Could you check a few things on this model? Use its own coordinates, in mm. Face numbers are marked on the shaded views. A direction names the side the tool comes from. Give positions to 0.01 mm unless a question says otherwise; leave off trailing zeros. Write each loop counter-clockwise with the first axis right and the second up, starting at its lowest first coordinate (ties: lowest second). Pieces come first, ordered by that corner, then holes. Notation, with made-up numbers: M 36,22.5 L 84,22.5 A14 ccw 84,48.5 Z; hole C 60,69 d9. An arc over 180 degrees is marked long. Use one line per item in the form item = value.
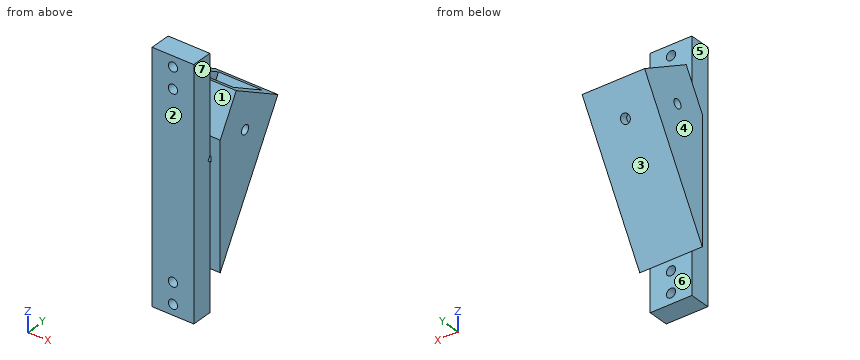
Autodesk Inventor part; units mm, degrees
ref_plane "YZ Plane" through (0, 0, 0) normal (1, 0, 0) x (0, 1, 0)
ref_plane "XZ Plane" through (0, 0, 0) normal (0, 1, 0) x (-1, 0, 0)
ref_plane "XY Plane" through (0, 0, 0) normal (0, 0, 1) x (1, 0, 0)
sketch "Sketch1" plane through (0, 0, 0) normal (1, 0, 0) x (0, 1, 0)
  line L0 (0, 0) -> (12.7, 21.997)
  line L1 (0, 0) -> (0, 47.397)
  line L2 (0, 0) -> (0, -101.6)
  line L3 (12.7, 21.997) -> (45.6956, 2.947)
  line L4 (45.6956, 2.947) -> (0, -76.2)
  line L5 (12.7, 21.997) -> (0, 21.997) construction
  line L6 (0, 47.397) -> (-12.7, 47.397)
  line L7 (-12.7, 47.397) -> (-12.7, -76.2)
  line L8 (0, -101.6) -> (-12.7, -101.6)
  line L9 (-12.7, -101.6) -> (-12.7, -76.2)
  dimension "d0" = 38.1
  dimension "d1" = 25.4
  dimension "d6" = 30
  dimension "d7" = 25.4
  dimension "d21" = 25.4
  dimension "d22" = 12.7
extrude "Extrusion2" add sketch "Sketch1" along normal mid plane 38.1 contours L0 L3 L4 L2
extrude "Extrusion3" add sketch "Sketch1" along normal mid plane 25.4
sketch "Sketch2" plane through (-19.05, 12.7, 21.997) normal (0, 0.5, 0.8660254) x (1, 0, 0)
  line L0 (32.385, 5.715) -> (32.385, 32.385)
  line L1 (32.385, 32.385) -> (5.715, 32.385)
  line L2 (5.715, 32.385) -> (5.715, 5.715)
  line L3 (5.715, 5.715) -> (32.385, 5.715)
  line L4 (32.385, 5.715) -> (5.715, 32.385) construction
  line L5 (32.385, 32.385) -> (5.715, 5.715) construction
  line L6 (0, 0) -> (0, 38.1)
  line L7 (38.1, 38.1) -> (38.1, 0)
  line L8 (0, 38.1) -> (38.1, 38.1)
  point P0 (19.05, 0)
  point P1 (19.05, 19.05)
  dimension "d16" = 26.67
  dimension "d17" = 19.05
  dimension "d18" = 19.05
extrude "Extrusion4" cut sketch "Sketch2" against normal blind 38.1
sketch "Sketch3" plane through (-12.7, 0, 47.397) normal (0, 1, 0) x (1, 0, 0)
  point P0 (12.7, 47.397)
sketch "Sketch4" plane through (-12.7, 0, 47.397) normal (0, 1, 0) x (1, 0, 0)
  line L0 (25.4, 0) -> (0, 0)
  line L1 (-6.35, 25.4) -> (31.75, 25.4)
  line L2 (0, 123.597) -> (25.4, 123.597)
  line L3 (25.4, 148.997) -> (0, 148.997)
  point P0 (12.7, 47.397)
  point P1 (12.7, 6.35)
  point P2 (12.7, 19.05)
  point P3 (12.7, 129.947)
  point P4 (12.7, 142.647)
  dimension "d23" = 6.35
  dimension "d24" = 6.35
  dimension "d25" = 6.35
  dimension "d26" = 6.35
hole "Hole1" at (0, 0, 41.047) at (0, 0, 28.347) at (0, 0, -82.55) at (0, 0, -95.25) direction (0, -1, 0) diameter 5.6134 end through all
sketch "Sketch5" plane through (19.05, 0, 0) normal (1, 0, 0) x (0, 0, -1)
  line L0 (-21.997, 12.7) -> (-2.947, 45.6956) construction
  line L1 (-12.472, 29.1978) -> (38.1, 0) construction
  line L2 (0, 0) -> (76.2, 0) construction
  line L3 (-21.997, 12.7) -> (0, 0) construction
  point P0 (4.0257, 19.6728)
  dimension "d34" = 19.05
sketch "Sketch6" plane through (-19.05, 45.6956, 2.947) normal (0, 0.8660254, -0.5) x (1, 0, 0)
  line L0 (0, 0) -> (38.1, 0)
  point P0 (19.05, 25.4)
  point P1 (19.05, 19.05)
  dimension "d35" = 19.05
hole "Hole2" at (0, 36.1706, -13.5507) direction (0, -0.8660254, 0.5) diameter 5.6134 depth 5.715
hole "Hole3" at (19.05, 19.6728, -4.0257) direction (-1, 0, 0) diameter 5.6134 end through all
properties part number "30degreeAttachement" material "PBT Plastic"
1) I want a section at C-C, the plane x = 0. Count the separate pieces of the cut face and the enclosed holes in it, plus the area to 3 significant figures.
Checked values:
separate_pieces = 6
enclosed_holes = 0
area = 2,780 mm2
2) I want a section at A-A, the plane z = -95.25. Please give me the cut outline in (x, y), plus the area to 3 significant figures.
Checked values:
outline = M -12.7,-12.7 L -2.81,-12.7 L -2.81,0 L -12.7,0 Z; M 2.81,-12.7 L 12.7,-12.7 L 12.7,0 L 2.81,0 Z
area = 251 mm2
3) For the marked faces 5, 6 and 7, which set-ups out of +Z, -Z, +X, -X, +Y, -Y let a thin tool reach every point of the face, with its end or its side?
Checked values:
face_5 = +Z, -Z, -X, -Y
face_6 = -Z, +X, -X, +Y
face_7 = +Z, -Z, +X, -Y
4) For pin 1 Ø5 at (x, z) = (-16, -26.5) entering from -Y; pin 2 Ø3 at (x, z) = (-13, -86) entering from +Y; pin 3 Ø2 at (x, y) = (-10, 6.5) entering from -Z; pin 4 Ø5 at (x, z) = (0, 41.047) entering from -Y, each with a flat end and sliding along its axis, tell me the tip position at first contact or that it passes through.
Checked values:
pin_1 = 0
pin_2 = 0
pin_3 = -66.67
pin_4 = through
5) If I drill on L1, parallel to Z at x = 0, y = -5.5; L2, parallel to X at y = 12.5, z = 6 (3 decimals); L3, parallel to Y at x = -12, z = 26, over which ranges is the centre line in solid material (lowest first)?
Checked values:
L1 = -101.6 to -98.06, -92.44 to -85.36, -79.74 to 25.54, 31.15 to 38.24, 43.85 to 47.4
L2 = -19.05 to -13.335, 13.335 to 19.05
L3 = -12.7 to 0
6) I want a section at D-D, the plane z = -31.5. Please give me the cut outline in (x, y).
Checked values:
outline = M -19.05,0 L -12.7,0 L -12.7,-12.7 L 12.7,-12.7 L 12.7,0 L 19.05,0 L 19.05,25.81 L -19.05,25.81 Z
7) I want a section at B-B, the plane x = -10. Please give me the cut outline in (y, z), plus the area to 3 significant figures.
Checked values:
outline = M -12.7,-101.6 L 0,-101.6 L 0,-76.2 L 45.7,2.95 L 40.75,5.8 L 21.7,-27.19 L -1.4,-13.86 L 17.65,19.14 L 12.7,22 L 0,0 L 0,47.4 L -12.7,47.4 Z
area = 3,100 mm2
8) Thinking about a two-plate mould opening in Y: for the marked faces 1, 2, 3 and 4, which applies, released by +Y, released by -Y, zero draft, split by the parting line, or undercut?
Checked values:
face_1 = undercut
face_2 = released by -Y
face_3 = released by +Y
face_4 = zero draft
